Read the model definition and answer for the solid it produces. Units are mm, in the model's axes. Face numbers are marked on the shaded views. A direction names the side the tool comes from. Give positions to 0.01 mm unless a question says otherwise; leave off trailing zeros. Order: outer loops, then holes, each group sorted by start corner. A loop starts at its lowest first (then second) coordinate and runs counter-clockwise, first axis right, second up. Notation, with made-up numbers: (67, 52.5) - (73, 52.5) arc R12 cw to (73, 56.5) - close; hole circle Ø7 at (62.5, -24). An arc over 180 degrees is marked (long way). Use a Markdown table: item, result. Add a question column.
1. A cutting plane is placed at A-A on y = 0. Determine the outline of the cut face in (x, z).
2. For a pull along X with two mould halves and no side action, classify the marked faces 1, 2, 3 and 4 as released by +X, released by -X, zero draft, split by the parting line, or undercut.
3. Flat-ended cylindrical pins translate along their axes: P1, Ø2, axis at y = -44.5, z = -14, coming from the +X side; P2, Ø2, axis at x = 45.5, z = -10, coming from the -Y side; P3, Ø5, axis at y = 46, z = -10, coming from the -X side; P4, Ø7, axis at x = -42.5, y = 42.5, coming from the -Z side. Find the tip coordinate at first contact, or state that the pin passes through.
4. Consider L1, parallel to Y at x = 0, z = 8; L2, parallel to Y at x = 42.5, z = -15; L3, parallel to Y at x = 42, z = 1. Determine where each line is inside the solid, lowest interval first.
5. A cutting plane is placed at C-C on z = 6.5. Determine the outline of the cut face in (x, y), and give its area (3 significant figures).
6. A cutting plane is placed at D-D on z = -10. State how many separate pieces and enclosed holes the cut face has, and give its area (3 significant figures).
7. Which of the six approach directions +Z, -Z, +X, -X, +Y, -Y give full straight-line access (tool end or side, diameter ignored) to the marked faces 5 and 6?
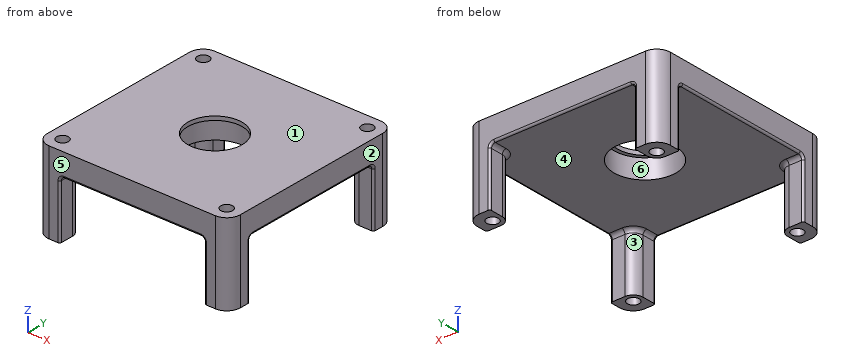
```python
from build123d import *

# Parameters (mm, degrees)
SKETCH2_W            = 100
SKETCH2_H            = 100
BOSS_EXTRUDE1_DEPTH  = 12
SKETCH3_R            = 16
CUT_EXTRUDE1_DEPTH   = 10
M6_CLEARANCE_HOLE1_D = 6.1
BOSS_EXTRUDE2_START  = 30
SKETCH17_R           = 3.05
BOSS_EXTRUDE2_DEPTH  = 30
CIRPATTERN1_COUNT    = 4
SKETCH18_R           = 14
CUT_EXTRUDE3_DEPTH   = 77.811457479
FILLET1_R            = 2
FILLET2_R            = 7
FILLET3_R            = 1


with BuildPart() as part:
    # Sketch2 → Boss-Extrude1 (new body)
    with BuildSketch(Plane.XY):
        Rectangle(SKETCH2_W, SKETCH2_H)
    extrude(amount=BOSS_EXTRUDE1_DEPTH)

    # Sketch3 → Cut-Extrude1 (cut)
    with BuildSketch(Plane(origin=(0, 0, 0), x_dir=(-1, 0, 0), z_dir=(0, 0, -1))):
        Circle(SKETCH3_R)
    extrude(amount=-CUT_EXTRUDE1_DEPTH, mode=Mode.SUBTRACT)

    # M6 Clearance Hole1 (through all)
    with Locations(Plane(origin=(0, 0, 12), x_dir=(-1, 0, 0), z_dir=(0, 0, 1))):
        with Locations((42.5, -42.5), (-42.5, 42.5), (-42.5, -42.5), (42.5, 42.5)):
            Hole(M6_CLEARANCE_HOLE1_D / 2)

    # Sketch17 → Boss-Extrude2 (add)
    with BuildSketch(Plane(origin=(0, 0, 0), x_dir=(-1, 0, 0), z_dir=(0, 0, -1)).offset(BOSS_EXTRUDE2_START)):
        with BuildLine():
            Line((-37.45, 42.5), (-37.45, 50))
            Line((-37.45, 50), (-50, 50))
            Line((-50, 50), (-50, 37.45))
            Line((-50, 37.45), (-42.5, 37.45))
            ThreePointArc((-42.5, 37.45), (-38.929110755, 38.929110755), (-37.45, 42.5))
        make_face()
        with Locations(Location((-42.5, 42.5, 0), (0, 0, 180))):
            Circle(SKETCH17_R, mode=Mode.SUBTRACT)
    boss_extrude2 = extrude(amount=-BOSS_EXTRUDE2_DEPTH)

    # CirPattern1: Boss-Extrude2 ×4 about axis
    cirpattern1_axis = Axis((0, 0, 0), (0, 0, 1))
    for i in range(1, CIRPATTERN1_COUNT):
        add(boss_extrude2.rotate(cirpattern1_axis, i * 360 / CIRPATTERN1_COUNT))

    # Sketch18 → Cut-Extrude3 (cut, through all)
    with BuildSketch(Plane(origin=(0, 0, 0), x_dir=(-1, 0, 0), z_dir=(0, 0, -1))):
        Circle(SKETCH18_R)
    extrude(amount=-CUT_EXTRUDE3_DEPTH, mode=Mode.SUBTRACT)

    # Fillet1
    fillet1_edges = [part.edges().sort_by_distance(p)[0] for p in [
        (38.929110755, 38.929110755, 0),
        (37.45, 46.25, 0),
        (46.25, 37.45, 0),
        (-38.929110755, 38.929110755, 0),
        (-46.25, 37.45, 0),
        (-37.45, 46.25, 0),
        (-38.929110755, -38.929110755, 0),
        (-37.45, -46.25, 0),
        (-46.25, -37.45, 0),
        (38.929110755, -38.929110755, 0),
        (46.25, -37.45, 0),
        (37.45, -46.25, 0),
    ]]
    fillet(fillet1_edges, radius=FILLET1_R)

    # Fillet2
    fillet2_edges = [part.edges().sort_by_distance(p)[0] for p in [
        (50, -50, -9),
        (-50, -50, -9),
        (-50, 50, -9),
        (50, 50, -9),
    ]]
    fillet(fillet2_edges, radius=FILLET2_R)

    # Fillet3
    fillet3_edges = [part.edges().sort_by_distance(p)[0] for p in [
        (50, 0, 0),
        (0, -50, 0),
        (-50, 0, 0),
        (0, 50, 0),
        (-36.864213562, 50, -0.585786438),
        (-50, 36.864213562, -0.585786438),
        (-50, -36.864213562, -0.585786438),
        (-36.864213562, -50, -0.585786438),
        (36.864213562, -50, -0.585786438),
        (50, -36.864213562, -0.585786438),
        (50, 36.864213562, -0.585786438),
        (36.864213562, 50, -0.585786438),
        (37.45, 50, -16),
        (50, 37.45, -16),
        (-50, 37.45, -16),
        (-37.45, 50, -16),
        (-37.45, -50, -16),
        (-50, -37.45, -16),
        (50, -37.45, -16),
        (37.45, -50, -16),
    ]]
    fillet(fillet3_edges, radius=FILLET3_R)


solid = part.part
```
Output values:
| question | item | result |
|---|---|---|
| 1 | outline | (-50, 1) arc R1 ccw to (-49, 0) - (-16, 0) - (-16, 10) - (-14, 10) - (-14, 12) - (-50, 12) - close; (14, 10) - (16, 10) - (16, 0) - (49, 0) arc R1 ccw to (50, 1) - (50, 12) - (14, 12) - close |
| 2 | face 1 | zero draft |
| 2 | face 2 | released by +X |
| 2 | face 3 | undercut |
| 2 | face 4 | undercut |
| 3 | P1 | x = 49.98 |
| 3 | P2 | y = -49.84 |
| 3 | P3 | x = -49.98 |
| 3 | P4 | z = -30 |
| 4 | L1 | -50 to -16, 16 to 50 |
| 4 | L2 | -50 to -45.55, -39.45 to -37.45, 37.45 to 39.45, 45.55 to 50 |
| 4 | L3 | -50 to -45.51, -39.49 to 39.49, 45.51 to 50 |
| 5 | outline | (-50, -43) arc R7 ccw to (-43, -50) - (43, -50) arc R7 ccw to (50, -43) - (50, 43) arc R7 ccw to (43, 50) - (-43, 50) arc R7 ccw to (-50, 43) - close; hole circle Ø6.1 at (-42.5, -42.5); hole circle Ø6.1 at (-42.5, 42.5); hole circle Ø32 at (0, 0); hole circle Ø6.1 at (42.5, -42.5); hole circle Ø6.1 at (42.5, 42.5) |
| 5 | area | 9,040 mm² |
| 6 | separate pieces | 4 |
| 6 | enclosed holes | 4 |
| 6 | area | 447 mm² |
| 7 | face 5 | +Z, -Z, +X, -X, -Y |
| 7 | face 6 | -Z |
